Geometry check sheet. Reference: drawing and pictorial views, mm from the part's lowest x, y, z. A direction names the side the tool comes from. Give positions to 0.01 mm unless a question says otherwise; leave off trailing zeros. Order: outer loops, then holes, each group sorted by start corner. A loop starts at its lowest first (then second) coordinate and runs counter-clockwise, first axis right, second up.
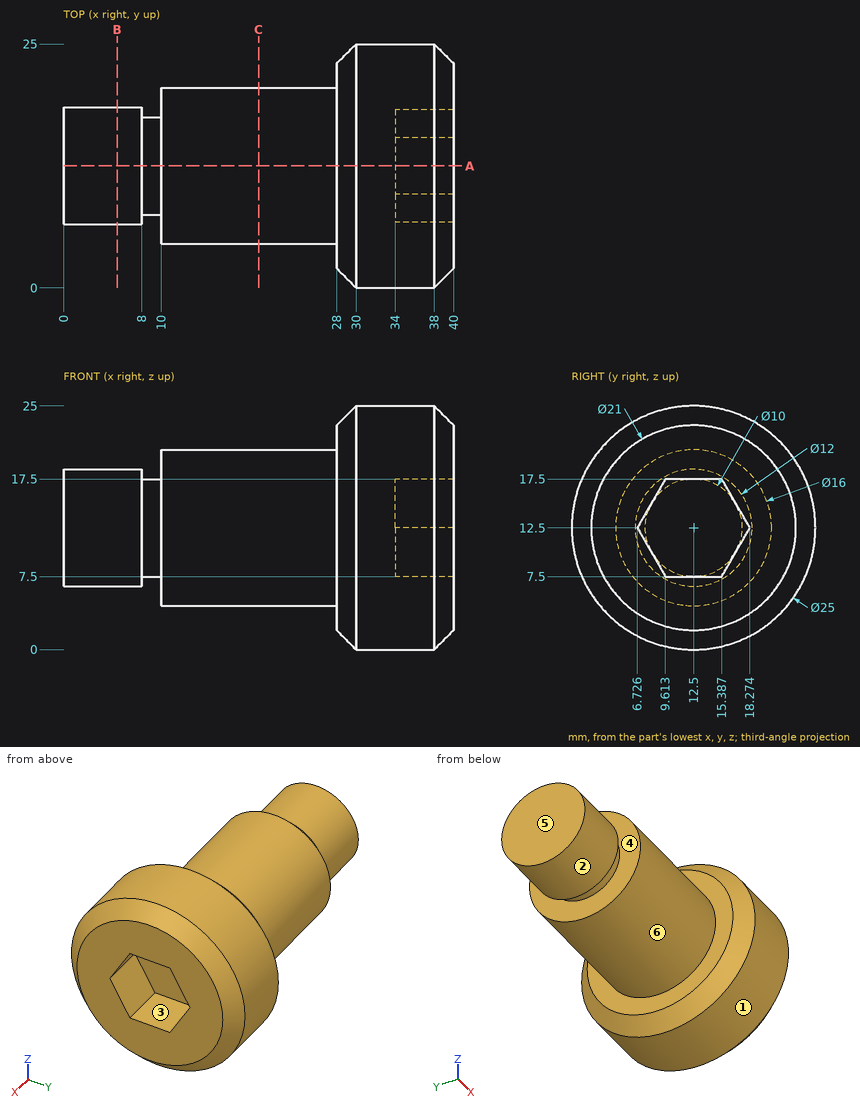
(1) Set-up check for the marked faces 1, 2 and 3: record each of +Z, -Z, +X, -X, +Y, -Y from which the full face is reachable in a straight line by a thin tool's end or side.
Response values:
face 1: +X, -X
face 2: -X
face 3: +X
(2) Cross-section at C-C on x = 20. Enter the section's corners in (y, z).
Response values:
outline: circle Ø16 at (12.5, 12.5)
(3) Gauge pin test, flat ends, axial feed: pin 1 Ø3 at (x, z) = (20, 7) entering from +Y; pin 2 Ø4 at (x, y) = (14, 4) entering from -Z (1 decimal); pin 3 Ø2 at (x, z) = (16, 2.5) entering from -Y; pin 4 Ø3 at (y, z) = (14, 11.5) entering from +X. Record the tip position at first contact, or that the pin passes through.
Response values:
pin 1: stops at y = 19.43
pin 2: stops at z = 7.8
pin 3: passes through
pin 4: stops at x = 34
(4) Cross-section at A-A on y = 12.5. Enter the section's corners in (x, z), then the cut area to 3 significant figures.
Response values:
outline: (0, 6.5) - (8, 6.5) - (8, 7.5) - (10, 7.5) - (10, 4.5) - (28, 4.5) - (28, 2) - (30, 0) - (38, 0) - (40, 2) - (40, 7.5) - (34, 7.5) - (34, 17.5) - (40, 17.5) - (40, 23) - (38, 25) - (30, 25) - (28, 23) - (28, 20.5) - (10, 20.5) - (10, 17.5) - (8, 17.5) - (8, 18.5) - (0, 18.5) - close
area: 636 mm2
(5) Material ranges on L1, parallel to X at y = 9.5, z = 17; L2, parallel to X at y = 12.5, z = 10.25; L3, parallel to X at y = 11.5, z = 5.5, recorded low to high.
Response values:
L1: x = 0 to 8, 10 to 34
L2: x = 0 to 34
L3: x = 10 to 40
(6) Release check for a two-part mould opening along X. For the marked faces 4, 5 and 6 record: released by +X, released by -X, zero draft, split by the parting line, or undercut.
Response values:
face 4: undercut
face 5: released by -X
face 6: zero draft
(7) Cross-section at B-B on x = 5.5. Enter the section's corners in (y, z).
Response values:
outline: circle Ø12 at (12.5, 12.5)
